Input: part model. Units: mm. Frame: model coordinates. A direction names the side the tool comes from. Coordinates: 2 decimals unless noted, no trailing zeros. Write each loop counter-clockwise with the first axis right and the second up, starting at its lowest first coordinate (ties: lowest second). Pieces come first, ordered by that corner, then holes.
from build123d import *

# Parameters (mm, degrees)
SKETCH1_R               = 457
BOSS_EXTRUDE1_DEPTH     = 25
SKETCH2_R               = 350
BOSS_EXTRUDE2_DEPTH     = 25
CUT_EXTRUDE3_DEPTH      = 649.226812158
CUT_EXTRUDE3_DEPTH_BACK = 649.226812158
SKETCH3_R               = 25
SKETCH3_R_2             = 264


with BuildPart() as part:
    # Sketch1 → Boss-Extrude1 (new body)
    with BuildSketch(Plane.XY):
        Circle(SKETCH1_R)
    extrude(amount=BOSS_EXTRUDE1_DEPTH)

    # Sketch2 → Boss-Extrude2 (add)
    with BuildSketch(Plane.XY.offset(25)):
        Circle(SKETCH2_R)
    extrude(amount=BOSS_EXTRUDE2_DEPTH)

    # Sketch3 → Cut-Extrude3 (cut, two sides: drawn at the far end of the back side and taken through both)
    with BuildSketch(Plane.XY.offset(50).offset(-CUT_EXTRUDE3_DEPTH_BACK)):
        with Locations((0, 300)):
            Circle(SKETCH3_R)
        with Locations((259.807621135, 150)):
            Circle(SKETCH3_R)
        with Locations((259.807621135, -150)):
            Circle(SKETCH3_R)
        with Locations((0, -300)):
            Circle(SKETCH3_R)
        with Locations((-259.807621135, -150)):
            Circle(SKETCH3_R)
        with Locations((-259.807621135, 150)):
            Circle(SKETCH3_R)
        Circle(SKETCH3_R_2)
    extrude(amount=CUT_EXTRUDE3_DEPTH + CUT_EXTRUDE3_DEPTH_BACK, mode=Mode.SUBTRACT)


solid = part.part
Item 1: Material intervals for line 1 (Y direction, x = 0, z = 21); line 2 (X direction, y = -150, z = 31); line 3 (Y direction, x = 274.5, z = 16), sorted ascending.
Item 2: Section query A-A, the plane y = 0. Return loops of the section in (x, z), then the cut area to 4 significant figures.
Item 3: Pin query (flat end, axial travel): pin 1 Ø5 at (x, z) = (161, 34) entering from -Y; pin 2 Ø4 at (x, z) = (-151, 12.5) entering from +Y; pin 3 Ø6 at (x, z) = (-200, 38.5) entering from +Y. Return the tip coordinate at first contact, or that it passes through.
Item 4: Pull-direction query (Y, two-part tool) for faces 3 (the face through (-3.255, -275.213, 24.65)), 4 (the face through (-99.069, -446.133, 12.325)), 5 (the face through (-131, -232, 50)); classes: released by +Y, released by -Y, zero draft, split by the parting line, or undercut.
Item 5: Access query for faces 1 (the face through (-104, -336, 25)), 2 (the face through (283.653, 157.509, 24.65)). Directions: +Z, -Z, +X, -X, +Y, -Y. A direction counts if a zero-diameter tool reaches every point of the face in a straight line with its end or side. Return the directions, or none.
Item 6: Section query D-D, the plane x = -92. Return loops of the section in (y, z), then the cut area to 3 significant figures.
Item 7: Section query B-B, the plane z = 14.5. Return loops of the section in (x, y).
Item 8: Section query C-C, the plane x = 0. Return loops of the section in (y, z).
The answers:
1. line 1: y = -457 to -325, -275 to -264, 264 to 275, 325 to 457
1. line 2: x = -316.23 to -284.81, -234.81 to -217.25, 217.25 to 234.81, 284.81 to 316.23
1. line 3: y = -365.37 to -170.23, -129.77 to 129.77, 170.23 to 365.37
2. outline: (-457, 0) - (-264, 0) - (-264, 50) - (-350, 50) - (-350, 25) - (-457, 25) - close; (264, 0) - (457, 0) - (457, 25) - (350, 25) - (350, 50) - (264, 50) - close
2. area: 13,950 mm2
3. pin 1: stops at y = -312.05
3. pin 2: stops at y = 432.03
3. pin 3: stops at y = 289.29
4. face 3: undercut
4. face 4: split by the parting line
4. face 5: zero draft
5. face 1: +Z
5. face 2: +Z, -Z
6. outline: (-447.64, 0) - (-247.45, 0) - (-247.45, 50) - (-337.69, 50) - (-337.69, 25) - (-447.64, 25) - close; (247.45, 0) - (447.64, 0) - (447.64, 25) - (337.69, 25) - (337.69, 50) - (247.45, 50) - close
6. area: 14,500 mm2
7. outline: circle Ø914 at (0, 0); hole circle Ø50 at (-259.81, -150); hole circle Ø50 at (-259.81, 150); hole circle Ø528 at (0, 0); hole circle Ø50 at (0, -300); hole circle Ø50 at (0, 300); hole circle Ø50 at (259.81, -150); hole circle Ø50 at (259.81, 150)
8. outline: (-457, 0) - (-325, 0) - (-325, 50) - (-350, 50) - (-350, 25) - (-457, 25) - close; (-275, 0) - (-264, 0) - (-264, 50) - (-275, 50) - close; (264, 0) - (275, 0) - (275, 50) - (264, 50) - close; (325, 0) - (457, 0) - (457, 25) - (350, 25) - (350, 50) - (325, 50) - close
